from build123d import *

# Parameters (mm, degrees)
BASE_FLANGE1_DEPTH = 300
CUT_EXTRUDE1_REACH = 303.544
SKETCH6_R          = 2.5


# Sheet-metal steps are written as plain solids
with BuildPart() as part:
    # Sketch1 → Base-Flange1 (new body)
    with BuildSketch(Plane(origin=(0, 0, 0), x_dir=(0, 0, -1), z_dir=(1, 0, 0))):
        with BuildLine():
            Line((-20, 10), (-6, 10))
            ThreePointArc((-6, 10), (-1.757359313, 8.242640687), (0, 4))
            Line((0, 4), (0, -7))
            ThreePointArc((0, -7), (0.878679656, -9.121320344), (3, -10))
            Line((3, -10), (20, -10))
            Line((20, -10), (20, -13))
            Line((20, -13), (3, -13))
            ThreePointArc((3, -13), (-1.242640687, -11.242640687), (-3, -7))
            Line((-3, -7), (-3, 4))
            ThreePointArc((-3, 4), (-3.878679656, 6.121320344), (-6, 7))
            Line((-6, 7), (-20, 7))
            Line((-20, 7), (-20, 10))
        make_face()
    extrude(amount=BASE_FLANGE1_DEPTH)

    # Sketch6 → Cut-Extrude1 (cut, up to next)
    with BuildSketch(Plane(origin=(0, 10, 0), x_dir=(1, 0, 0), z_dir=(0, 1, 0)), mode=Mode.PRIVATE) as cut_extrude1_sk1:
        with Locations(Location((25, -13, 0), (0, 0, 270))):
            Circle(SKETCH6_R)
    cut_extrude1_tool1 = extrude(cut_extrude1_sk1.sketch, amount=-CUT_EXTRUDE1_REACH, mode=Mode.PRIVATE) & part.part
    # Sketch6 → Cut-Extrude1 (cut, up to next)
    with BuildSketch(Plane(origin=(0, 10, 0), x_dir=(1, 0, 0), z_dir=(0, 1, 0)), mode=Mode.PRIVATE) as cut_extrude1_sk2:
        with Locations(Location((75, -13, 0), (0, 0, 270))):
            Circle(SKETCH6_R)
    cut_extrude1_tool2 = extrude(cut_extrude1_sk2.sketch, amount=-CUT_EXTRUDE1_REACH, mode=Mode.PRIVATE) & part.part
    # Sketch6 → Cut-Extrude1 (cut, up to next)
    with BuildSketch(Plane(origin=(0, 10, 0), x_dir=(1, 0, 0), z_dir=(0, 1, 0)), mode=Mode.PRIVATE) as cut_extrude1_sk3:
        with Locations(Location((125, -13, 0), (0, 0, 270))):
            Circle(SKETCH6_R)
    cut_extrude1_tool3 = extrude(cut_extrude1_sk3.sketch, amount=-CUT_EXTRUDE1_REACH, mode=Mode.PRIVATE) & part.part
    # Sketch6 → Cut-Extrude1 (cut, up to next)
    with BuildSketch(Plane(origin=(0, 10, 0), x_dir=(1, 0, 0), z_dir=(0, 1, 0)), mode=Mode.PRIVATE) as cut_extrude1_sk4:
        with Locations(Location((175, -13, 0), (0, 0, 270))):
            Circle(SKETCH6_R)
    cut_extrude1_tool4 = extrude(cut_extrude1_sk4.sketch, amount=-CUT_EXTRUDE1_REACH, mode=Mode.PRIVATE) & part.part
    # Sketch6 → Cut-Extrude1 (cut, up to next)
    with BuildSketch(Plane(origin=(0, 10, 0), x_dir=(1, 0, 0), z_dir=(0, 1, 0)), mode=Mode.PRIVATE) as cut_extrude1_sk5:
        with Locations(Location((225, -13, 0), (0, 0, 270))):
            Circle(SKETCH6_R)
    cut_extrude1_tool5 = extrude(cut_extrude1_sk5.sketch, amount=-CUT_EXTRUDE1_REACH, mode=Mode.PRIVATE) & part.part
    # Sketch6 → Cut-Extrude1 (cut, up to next)
    with BuildSketch(Plane(origin=(0, 10, 0), x_dir=(1, 0, 0), z_dir=(0, 1, 0)), mode=Mode.PRIVATE) as cut_extrude1_sk6:
        with Locations(Location((275, -13, 0), (0, 0, 270))):
            Circle(SKETCH6_R)
    cut_extrude1_tool6 = extrude(cut_extrude1_sk6.sketch, amount=-CUT_EXTRUDE1_REACH, mode=Mode.PRIVATE) & part.part
    # Sketch6 → Cut-Extrude1 (cut, up to next)
    with BuildSketch(Plane(origin=(0, 10, 0), x_dir=(1, 0, 0), z_dir=(0, 1, 0)), mode=Mode.PRIVATE) as cut_extrude1_sk7:
        with Locations(Location((75, 11.5, 0), (0, 0, 270))):
            Circle(SKETCH6_R)
    cut_extrude1_tool7 = extrude(cut_extrude1_sk7.sketch, amount=-CUT_EXTRUDE1_REACH, mode=Mode.PRIVATE) & part.part
    # Sketch6 → Cut-Extrude1 (cut, up to next)
    with BuildSketch(Plane(origin=(0, 10, 0), x_dir=(1, 0, 0), z_dir=(0, 1, 0)), mode=Mode.PRIVATE) as cut_extrude1_sk8:
        with Locations(Location((125, 11.5, 0), (0, 0, 270))):
            Circle(SKETCH6_R)
    cut_extrude1_tool8 = extrude(cut_extrude1_sk8.sketch, amount=-CUT_EXTRUDE1_REACH, mode=Mode.PRIVATE) & part.part
    # Sketch6 → Cut-Extrude1 (cut, up to next)
    with BuildSketch(Plane(origin=(0, 10, 0), x_dir=(1, 0, 0), z_dir=(0, 1, 0)), mode=Mode.PRIVATE) as cut_extrude1_sk9:
        with Locations(Location((175, 11.5, 0), (0, 0, 270))):
            Circle(SKETCH6_R)
    cut_extrude1_tool9 = extrude(cut_extrude1_sk9.sketch, amount=-CUT_EXTRUDE1_REACH, mode=Mode.PRIVATE) & part.part
    # Sketch6 → Cut-Extrude1 (cut, up to next)
    with BuildSketch(Plane(origin=(0, 10, 0), x_dir=(1, 0, 0), z_dir=(0, 1, 0)), mode=Mode.PRIVATE) as cut_extrude1_sk10:
        with Locations(Location((225, 11.5, 0), (0, 0, 270))):
            Circle(SKETCH6_R)
    cut_extrude1_tool10 = extrude(cut_extrude1_sk10.sketch, amount=-CUT_EXTRUDE1_REACH, mode=Mode.PRIVATE) & part.part
    # Sketch6 → Cut-Extrude1 (cut, up to next)
    with BuildSketch(Plane(origin=(0, 10, 0), x_dir=(1, 0, 0), z_dir=(0, 1, 0)), mode=Mode.PRIVATE) as cut_extrude1_sk11:
        with Locations(Location((275, 11.5, 0), (0, 0, 270))):
            Circle(SKETCH6_R)
    cut_extrude1_tool11 = extrude(cut_extrude1_sk11.sketch, amount=-CUT_EXTRUDE1_REACH, mode=Mode.PRIVATE) & part.part
    # Sketch6 → Cut-Extrude1 (cut, up to next)
    with BuildSketch(Plane(origin=(0, 10, 0), x_dir=(1, 0, 0), z_dir=(0, 1, 0)), mode=Mode.PRIVATE) as cut_extrude1_sk12:
        with Locations(Location((25, 11.5, 0), (0, 0, 270))):
            Circle(SKETCH6_R)
    cut_extrude1_tool12 = extrude(cut_extrude1_sk12.sketch, amount=-CUT_EXTRUDE1_REACH, mode=Mode.PRIVATE) & part.part
    add(cut_extrude1_tool1.solids().sort_by_distance((25, 10, 13))[0], mode=Mode.SUBTRACT)
    add(cut_extrude1_tool2.solids().sort_by_distance((75, 10, 13))[0], mode=Mode.SUBTRACT)
    add(cut_extrude1_tool3.solids().sort_by_distance((125, 10, 13))[0], mode=Mode.SUBTRACT)
    add(cut_extrude1_tool4.solids().sort_by_distance((175, 10, 13))[0], mode=Mode.SUBTRACT)
    add(cut_extrude1_tool5.solids().sort_by_distance((225, 10, 13))[0], mode=Mode.SUBTRACT)
    add(cut_extrude1_tool6.solids().sort_by_distance((275, 10, 13))[0], mode=Mode.SUBTRACT)
    add(cut_extrude1_tool7.solids().sort_by_distance((75, 10, -11.5))[0], mode=Mode.SUBTRACT)
    add(cut_extrude1_tool8.solids().sort_by_distance((125, 10, -11.5))[0], mode=Mode.SUBTRACT)
    add(cut_extrude1_tool9.solids().sort_by_distance((175, 10, -11.5))[0], mode=Mode.SUBTRACT)
    add(cut_extrude1_tool10.solids().sort_by_distance((225, 10, -11.5))[0], mode=Mode.SUBTRACT)
    add(cut_extrude1_tool11.solids().sort_by_distance((275, 10, -11.5))[0], mode=Mode.SUBTRACT)
    add(cut_extrude1_tool12.solids().sort_by_distance((25, 10, -11.5))[0], mode=Mode.SUBTRACT)


solid = part.part
Read the model definition and answer for the solid it produces. Units are mm, in the model's axes. A direction names the side the tool comes from. Coordinates: 2 decimals unless noted, no trailing zeros. Loops run counter-clockwise (first coordinate to the right, second up) from the corner with the lowest first, then second, coordinate; pieces in that order, holes last.
Q1. Which of the six approach directions +Z, -Z, +X, -X, +Y, -Y give full straight-line access (tool end or side, diameter ignored) to faces 5 (the face through (148, 7, 13)), 6 (the face through (148, -13, -12)), 7 (the face through (148, -1, 0))?
Q2. The part is cut by section A-A on z = -11.5. Write down the section's boundary in (x, y), and give its area (3 significant figures).
Q3. The part is cut by section B-B on x = 275. Write down the section's boundary in (y, z), and give its area (3 significant figures).
Q4. The part is cut by section D-D on y = -3. Write down the section's boundary in (x, z).
Q5. The mould has two halves that part along X. Classify faces 1 (the face through (148, 10, 13)), 2 (the face through (27.48, -11.48, -11.83)), 3 (the face through (300, -1, 1)), 4 (the face through (0, -1, 1)): +X half, -X half, draft (parallel to the pull), parting line (faces both ways), or undercut.
Q6. Consider probe 1 along Z at (x, y) = (226, 0.5); probe 2 along Y at (x, z) = (116.5, -14); probe 3 along Y at (x, z) = (50, 7). Determine where each line is inside the solid, lowest interval first.
Q7. Each of these flat-tipped pins is pushed along its axis until it touches: pin 1 Ø11 at (x, z) = (180, 15.5) entering from -Y; pin 2 Ø8 at (x, z) = (225, -11.5) entering from +Y; pin 3 Ø12 at (x, y) = (142, 0.5) entering from -Z; pin 4 Ø8 at (y, z) = (7.5, -5.5) entering from -X. Where does it stop, or does it pass through?
Q8. The part is cut by section C-C on x = 153. Write down the section's boundary in (y, z).
Results below:
1. face 5: +Z, +X, -X, -Y
1. face 6: +Z, -Z, +X, -X, -Y
1. face 7: -Z, +X, -X, +Y
2. outline: (0, -13) - (22.5, -13) - (22.5, -10) - (0, -10) - close; (27.5, -13) - (72.5, -13) - (72.5, -10) - (27.5, -10) - close; (77.5, -13) - (122.5, -13) - (122.5, -10) - (77.5, -10) - close; (127.5, -13) - (172.5, -13) - (172.5, -10) - (127.5, -10) - close; (177.5, -13) - (222.5, -13) - (222.5, -10) - (177.5, -10) - close; (227.5, -13) - (272.5, -13) - (272.5, -10) - (227.5, -10) - close; (277.5, -13) - (300, -13) - (300, -10) - (277.5, -10) - close
2. area: 810 mm2
3. outline: (-13, -20) - (-10, -20) - (-10, -14) - (-13, -14) - close; (-13, -9) - (-10, -9) - (-10, -3) arc R3 cw to (-7, 0) - (4, 0) arc R6 ccw to (10, 6) - (10, 10.5) - (7, 10.5) - (7, 6) arc R3 cw to (4, 3) - (-7, 3) arc R6 ccw to (-13, -3) - close; (7, 15.5) - (10, 15.5) - (10, 20) - (7, 20) - close
3. area: 138 mm2
4. outline: (0, 0) - (300, 0) - (300, 3) - (0, 3) - close
5. face 1: draft
5. face 2: undercut
5. face 3: +X half
5. face 4: -X half
6. probe 1: z = 0 to 3
6. probe 2: y = -13 to -10
6. probe 3: y = 7 to 10
7. pin 1: stops at y = 7
7. pin 2: stops at y = -10
7. pin 3: stops at z = 0
7. pin 4: passes through
8. outline: (-13, -20) - (-10, -20) - (-10, -3) arc R3 cw to (-7, 0) - (4, 0) arc R6 ccw to (10, 6) - (10, 20) - (7, 20) - (7, 6) arc R3 cw to (4, 3) - (-7, 3) arc R6 ccw to (-13, -3) - close
